Read the model definition and answer for the solid it produces. Units are mm, in the model's axes. Face numbers are marked on the shaded views. Give positions to 0.01 mm unless a question says otherwise; leave off trailing zeros. Loops run counter-clockwise (first coordinate to the right, second up) from the corner with the lowest first, then second, coordinate; pieces in that order, holes last. Notation, with made-up numbers: (-36, -29) - (18, -29) arc R18 ccw to (18, -25) - close; hole circle Ø10 at (-28.5, -32.75). An arc over 180 degrees is marked (long way). Put each result on its own line as item: value. Start each with the question number.
1. A cutting plane is placed at D-D, the plane z = 29.5. Determine the outline of the cut face in (x, y).
2. A cutting plane is placed at A-A, the plane y = 0. Determine the outline of the cut face in (x, z), plus the area to 3 significant figures.
3. A cutting plane is placed at B-B, the plane x = 0. Determine the outline of the cut face in (y, z).
4. Consider L1, parallel to X at y = 1.5, z = 101.5; L2, parallel to Y at x = 2, z = 82.5; L3, parallel to Z at x = 0, y = 104. Determine where each line is inside the solid, lowest interval first. Write a range as from..to.
5. For a pull along X with two mould halves and no side action, classify the marked faces 1, 2 and 3 as released by +X, released by -X, zero draft, split by the parting line, or undercut.
6. A cutting plane is placed at C-C, the plane x = 56. Determine the outline of the cut face in (y, z), plus the area to 3 significant figures.
7. Given pin 1 Ø4 at (x, z) = (26, 159) entering from -Y; pin 2 Ø1 at (x, z) = (14.5, 212) entering from +Y; pin 3 Ø8 at (x, z) = (-61, 106) entering from +Y, each flat-ended and moving along its own axis, determine where each tip first touches the part or whether it passes through.
Autodesk Inventor part; units mm, degrees
ref_plane "YZ Plane" through (0, 0, 0) normal (1, 0, 0) x (0, 1, 0)
ref_plane "XZ Plane" through (0, 0, 0) normal (0, 1, 0) x (-1, 0, 0)
ref_plane "XY Plane" through (0, 0, 0) normal (0, 0, 1) x (1, 0, 0)
sketch "Sketch1" plane through (0, 0, 0) normal (0, 0, 1) x (1, 0, 0)
  circle A0 centre (0, 0) radius 99.6
  circle A1 centre (0, 0) radius 107.6
  dimension "d0" = 199.2
  dimension "d1" = 8
extrude "Extrusion1" add sketch "Sketch1" along normal blind 254
sketch "Sketch3" plane through (0, 0, 0) normal (0, 0, -1) x (-1, 0, 0)
  circle A0 centre (0, 0) radius 107.6 construction
  circle A1 centre (0, 0) radius 99.6 construction
  arc A2 (-43.4971, -89.6) -> (43.4971, -89.6) centre (0, 0) ccw
  line L0 (0, -99.6) -> (0, -89.6) construction
  line L1 (43.4971, -89.6) -> (-43.4971, -89.6)
  dimension "d11" = 10
extrude "Extrusion3" add sketch "Sketch3" against normal up to surface (254 mm away)
sketch "Sketch4" plane through (0, 0, 0) normal (0, 1, 0) x (-1, 0, 0)
  circle A0 centre (0, 154) radius 7.5
  line L0 (107.6, 254) -> (-107.6, 254) construction
  line L1 (107.6, 0) -> (-107.6, 0) construction
  point P0 (0, 0)
  point P1 (0, 0)
  dimension "d14" = 15
  dimension "d15" = 100
extrude "Extrusion4" cut sketch "Sketch4" along normal up to surface
properties part number "FrontTubeV1_3DPrint"
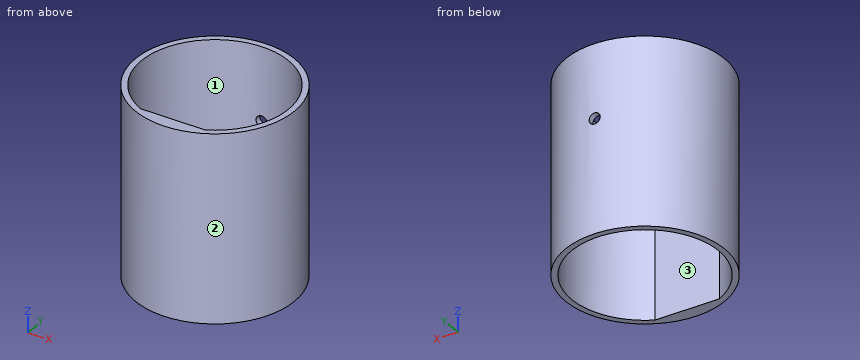
Return value:
1. outline: circle Ø215.2 at (0, 0); hole (-43.5, -89.6) - (43.5, -89.6) arc R99.6 ccw (long way) to start
2. outline: (-107.6, 0) - (-99.6, 0) - (-99.6, 254) - (-107.6, 254) - close; (99.6, 0) - (107.6, 0) - (107.6, 254) - (99.6, 254) - close
2. area: 4,060 mm2
3. outline: (-107.6, 0) - (-89.6, 0) - (-89.6, 254) - (-107.6, 254) - close; (99.6, 0) - (107.6, 0) - (107.6, 146.5) - (99.6, 146.5) - close; (99.6, 161.5) - (107.6, 161.5) - (107.6, 254) - (99.6, 254) - close
4. L1: x = -107.59..-99.59, 99.59..107.59
4. L2: y = -107.58..-89.6, 99.58..107.58
4. L3: z = 0..146.5, 161.5..254
5. face 1: undercut
5. face 2: split by the parting line
5. face 3: undercut
6. outline: (-91.88, 0) - (-82.37, 0) - (-82.37, 254) - (-91.88, 254) - close; (82.37, 0) - (91.88, 0) - (91.88, 254) - (82.37, 254) - close
6. area: 4,830 mm2
7. pin 1: stops at y = -104.89
7. pin 2: stops at y = 106.69
7. pin 3: stops at y = 91.26
